Geometry: final body of the model. Coordinates: model frame, mm. A direction names the side the tool comes from. Round coordinates to 2 decimals unless told otherwise and drop trailing zeros. Write each loop counter-clockwise with the first axis right and the second up, starting at its lowest first coordinate (ties: lowest second). Pieces come first, ordered by that corner, then holes. Notation, with made-up numbers: (-24.5, 85) -> (-6.5, 85) arc R28 cw to (-6.5, 116) -> close; hole circle Ø6 at (31, 16). An arc over 180 degrees is marked (long way). One line per item, written item: value. Start each with the question number.
from build123d import *

# Parameters (mm, degrees)
F1_DEPTH = 50.8
F2_W     = 8.89
F2_H     = 8.255
F3_DEPTH = 38.1
F4_R     = 3.3655
F4_R_2   = 2.0955
F5_DEPTH = 2.54
F6_DEPTH = 53.34


with BuildPart() as f1:
    # F0 (on Top) → F1 (new body)
    with BuildSketch(Plane.XY):
        with BuildLine():
            Line((-27.305, 3.3655), (-27.305, 4.9141779831))
            ThreePointArc((-27.305, 4.9141779831), (-29.1268062902, -3.7268062902), (-20.4858220169, -1.905))
            Line((-20.4858220169, -1.905), (-22.0345, -1.905))
            Line((-22.0345, -1.905), (-22.0345, 0))
            ThreePointArc((-22.0345, 0), (-27.7797678721, -2.3797678721), (-25.4, 3.3655))
            Line((-25.4, 3.3655), (-27.305, 3.3655))
        make_face()
        with BuildLine():
            ThreePointArc((-23.495, 35.7206557626), (-25.4, 35.052), (-27.305, 35.7206557626))
            Line((-27.305, 35.7206557626), (-27.305, 4.9141779831))
            ThreePointArc((-27.305, 4.9141779831), (-25.4, 5.2705), (-23.495, 4.9141779831))
            Line((-23.495, 4.9141779831), (-23.495, 35.7206557626))
        make_face()
        with BuildLine():
            ThreePointArc((-23.495, 4.9141779831), (-25.4, 5.2705), (-27.305, 4.9141779831))
            Line((-27.305, 4.9141779831), (-27.305, 3.3655))
            Line((-27.305, 3.3655), (-25.4, 3.3655))
            Line((-25.4, 3.3655), (-23.495, 3.3655))
            Line((-23.495, 3.3655), (-23.495, 4.9141779831))
        make_face()
        with BuildLine():
            Line((-22.0345, -1.905), (-20.4858220169, -1.905))
            ThreePointArc((-20.4858220169, -1.905), (-20.2193463101, -0.9690188826), (-20.1295, 0))
            ThreePointArc((-20.1295, 0), (-20.2193463101, 0.9690188826), (-20.4858220169, 1.905))
            Line((-20.4858220169, 1.905), (-22.0345, 1.905))
            Line((-22.0345, 1.905), (-22.0345, 0))
            Line((-22.0345, 0), (-22.0345, -1.905))
        make_face()
        with BuildLine():
            ThreePointArc((-20.4858220169, 1.905), (-21.6731937098, 3.7268062902), (-23.495, 4.9141779831))
            Line((-23.495, 4.9141779831), (-23.495, 3.3655))
            Line((-23.495, 3.3655), (-25.4, 3.3655))
            ThreePointArc((-25.4, 3.3655), (-23.0202321279, 2.3797678721), (-22.0345, 0))
            Line((-22.0345, 0), (-22.0345, 1.905))
            Line((-22.0345, 1.905), (-20.4858220169, 1.905))
        make_face()
        with BuildLine():
            ThreePointArc((-20.1295, 0), (-20.2193463101, -0.9690188826), (-20.4858220169, -1.905))
            Line((-20.4858220169, -1.905), (0, -1.905))
            Line((0, -1.905), (0, 0))
            Line((0, 0), (0, 1.905))
            Line((0, 1.905), (-20.4858220169, 1.905))
            ThreePointArc((-20.4858220169, 1.905), (-20.2193463101, 0.9690188826), (-20.1295, 0))
        make_face()
        with BuildLine():
            Line((20.4858220169, 1.905), (0, 1.905))
            Line((0, 1.905), (0, 0))
            Line((0, 0), (20.1295, 0))
            ThreePointArc((20.1295, 0), (20.2193463101, 0.9690188826), (20.4858220169, 1.905))
        make_face()
        with BuildLine():
            Line((22.0345, 1.905), (20.4858220169, 1.905))
            ThreePointArc((20.4858220169, 1.905), (20.2193463101, 0.9690188826), (20.1295, 0))
            Line((20.1295, 0), (22.0345, 0))
            Line((22.0345, 0), (22.0345, 1.905))
        make_face()
        with BuildLine():
            Line((22.0345, -1.905), (20.4858220169, -1.905))
            ThreePointArc((20.4858220169, -1.905), (26.3690188826, -5.1806536899), (30.6705, 0))
            ThreePointArc((30.6705, 0), (29.7484751782, 2.9780755321), (27.305, 4.9141779831))
            Line((27.305, 4.9141779831), (27.305, 3.3655))
            Line((27.305, 3.3655), (25.4, 3.3655))
            ThreePointArc((25.4, 3.3655), (27.7797678721, 2.3797678721), (28.7655, 0))
            ThreePointArc((28.7655, 0), (25.4, -3.3655), (22.0345, 0))
            Line((22.0345, 0), (22.0345, -1.905))
        make_face()
        with BuildLine():
            ThreePointArc((20.1295, 0), (20.2193463101, -0.9690188826), (20.4858220169, -1.905))
            Line((20.4858220169, -1.905), (22.0345, -1.905))
            Line((22.0345, -1.905), (22.0345, 0))
            Line((22.0345, 0), (20.1295, 0))
        make_face()
        with BuildLine():
            Line((0, 0), (0, -1.905))
            Line((0, -1.905), (20.4858220169, -1.905))
            ThreePointArc((20.4858220169, -1.905), (20.2193463101, -0.9690188826), (20.1295, 0))
            Line((20.1295, 0), (0, 0))
        make_face()
        with BuildLine():
            Line((27.305, 3.3655), (27.305, 4.9141779831))
            ThreePointArc((27.305, 4.9141779831), (26.3690188826, 5.1806536899), (25.4, 5.2705))
            Line((25.4, 5.2705), (25.4, 3.3655))
            Line((25.4, 3.3655), (27.305, 3.3655))
        make_face()
        with BuildLine():
            ThreePointArc((25.4, 5.2705), (26.3690188826, 5.1806536899), (27.305, 4.9141779831))
            Line((27.305, 4.9141779831), (27.305, 35.7206557626))
            ThreePointArc((27.305, 35.7206557626), (26.4094708427, 35.2240179733), (25.4, 35.052))
            Line((25.4, 35.052), (25.4, 5.2705))
        make_face()
        with BuildLine():
            Line((23.495, 35.7206557626), (23.495, 4.9141779831))
            ThreePointArc((23.495, 4.9141779831), (24.4309811174, 5.1806536899), (25.4, 5.2705))
            Line((25.4, 5.2705), (25.4, 35.052))
            ThreePointArc((25.4, 35.052), (24.3905291573, 35.2240179733), (23.495, 35.7206557626))
        make_face()
        with BuildLine():
            ThreePointArc((25.4, 5.2705), (24.4309811174, 5.1806536899), (23.495, 4.9141779831))
            Line((23.495, 4.9141779831), (23.495, 3.3655))
            Line((23.495, 3.3655), (25.4, 3.3655))
            Line((25.4, 3.3655), (25.4, 5.2705))
        make_face()
        with BuildLine():
            ThreePointArc((23.495, 4.9141779831), (21.6731937098, 3.7268062902), (20.4858220169, 1.905))
            Line((20.4858220169, 1.905), (22.0345, 1.905))
            Line((22.0345, 1.905), (22.0345, 0))
            ThreePointArc((22.0345, 0), (23.0202321279, 2.3797678721), (25.4, 3.3655))
            Line((25.4, 3.3655), (23.495, 3.3655))
            Line((23.495, 3.3655), (23.495, 4.9141779831))
        make_face()
    extrude(amount=F1_DEPTH)

    # F2 (on Right) → F3 (cut, symmetric)
    with BuildSketch(Plane.YZ):
        with Locations((31.2756557626, 4.1275)):
            Rectangle(F2_W, F2_H)
        with BuildLine():
            Line((4.9141779831, 50.8), (4.9141779831, 30.582289685))
            add(Edge.make_bspline(
                [(4.9141779831, 30.582289685), (16.0486069147, 30.9902963569), (19.3334478065, 33.025734419), (35.7206557626, 43.18)],
                knots=[8.6020682106, 8.6020682106, 8.6020682106, 8.6020682106, 42.9134576882, 42.9134576882, 42.9134576882, 42.9134576882], degree=3))
            Line((35.7206557626, 43.18), (35.7206557626, 50.8))
            Line((35.7206557626, 50.8), (4.9141779831, 50.8))
        make_face()
        with BuildLine():
            add(Edge.make_bspline(
                [(-5.2705, 30.48), (-1.1621300748, 30.48), (2.1227108169, 30.48), (4.9141779831, 30.582289685)],
                knots=[0, 0, 0, 0, 8.6020682106, 8.6020682106, 8.6020682106, 8.6020682106], degree=3))
            Line((4.9141779831, 30.582289685), (4.9141779831, 50.8))
            Line((4.9141779831, 50.8), (-5.2705, 50.8))
            Line((-5.2705, 50.8), (-5.2705, 30.48))
        make_face()
    extrude(amount=F3_DEPTH, both=True, mode=Mode.SUBTRACT)

    # F4 (on face) → F5 (join)
    with BuildSketch(Plane(origin=(0, 0, 0), x_dir=(1, 0, 0), z_dir=(0, 0, -1))):
        with Locations((-25.4, 0)):
            Circle(F4_R)
        with Locations((-25.4, 0)):
            Circle(F4_R_2, mode=Mode.SUBTRACT)
        with BuildLine():
            ThreePointArc((30.6705, 0), (26.3690188826, 5.1806536899), (20.4858220169, 1.905))
            ThreePointArc((20.4858220169, 1.905), (20.1295, 0), (20.4858220169, -1.905))
            ThreePointArc((20.4858220169, -1.905), (21.6731937098, -3.7268062902), (23.495, -4.9141779831))
            ThreePointArc((23.495, -4.9141779831), (25.4, -5.2705), (27.305, -4.9141779831))
            ThreePointArc((27.305, -4.9141779831), (29.7484751782, -2.9780755321), (30.6705, 0))
        make_face()
        with Locations((25.4, 0)):
            Circle(F4_R, mode=Mode.SUBTRACT)
        with Locations((25.4, 0)):
            Circle(F4_R)
        with Locations((25.4, 0)):
            Circle(F4_R_2, mode=Mode.SUBTRACT)
    extrude(amount=-F5_DEPTH)

    # F0 (on Top) → F6 (join)
    with BuildSketch(Plane.XY):
        with BuildLine():
            Line((-27.305, 38.1), (-27.305, 35.7206557626))
            ThreePointArc((-27.305, 35.7206557626), (-25.4, 35.052), (-23.495, 35.7206557626))
            Line((-23.495, 35.7206557626), (-23.495, 38.1))
            Line((-23.495, 38.1), (-27.305, 38.1))
        make_face()
        with BuildLine():
            ThreePointArc((-23.495, 35.7206557626), (-22.6525699281, 36.7801772846), (-22.352, 38.1))
            ThreePointArc((-22.352, 38.1), (-26.7198227154, 40.8474300719), (-27.305, 35.7206557626))
            Line((-27.305, 35.7206557626), (-27.305, 38.1))
            Line((-27.305, 38.1), (-23.495, 38.1))
            Line((-23.495, 38.1), (-23.495, 35.7206557626))
        make_face()
        with BuildLine():
            ThreePointArc((28.448, 38.1), (24.0801772846, 40.8474300719), (23.495, 35.7206557626))
            Line((23.495, 35.7206557626), (23.495, 38.1))
            Line((23.495, 38.1), (25.4, 38.1))
            Line((25.4, 38.1), (27.305, 38.1))
            Line((27.305, 38.1), (27.305, 35.7206557626))
            ThreePointArc((27.305, 35.7206557626), (28.1474300719, 36.7801772846), (28.448, 38.1))
        make_face()
        with BuildLine():
            ThreePointArc((25.4, 35.052), (26.4094708427, 35.2240179733), (27.305, 35.7206557626))
            Line((27.305, 35.7206557626), (27.305, 38.1))
            Line((27.305, 38.1), (25.4, 38.1))
            Line((25.4, 38.1), (25.4, 35.052))
        make_face()
        with BuildLine():
            Line((23.495, 38.1), (23.495, 35.7206557626))
            ThreePointArc((23.495, 35.7206557626), (24.3905291573, 35.2240179733), (25.4, 35.052))
            Line((25.4, 35.052), (25.4, 38.1))
            Line((25.4, 38.1), (23.495, 38.1))
        make_face()
    extrude(amount=F6_DEPTH)


solid = f1.part
(1) Section query A-A (z = 11). Output: boundary loops of the cut face in (x, y) (1 decimal), and give its area (3 significant figures).
(2) Pull-direction query (Y, two-part tool) for faces 1 (the face through (4, 1, 0)), 2 (the face through (-25, 31, 8.255)), 3 (the face through (23.495, 21, 21)), 4 (the face through (0, -1.905, 15)); classes: pulls with the +Y half, pulls with the -Y half, needs draft (parallel to the pull), parting line crosses it, or undercut.
(3) Line query: probe 1 along X at (y, z) = (0, 0.9); probe 2 along Y at (x, z) = (-25.4, 1.7); probe 3 along X at (y, z) = (0, 14). Output: solid intervals per line, ascending.
(4) Set-up query: faces 5 (the face through (27, -2, 2.54)), 6 (the face through (27.305, 20, 21)), 7 (the face through (25, 26.831, 4)). Return all of +Z, -Z, +X, -X, +Y, -Y with unobstructed straight access to the full face (end or side cutting, diameter ignored); none if empty.
(5) Section query B-B (y = 36.5). Output: boundary loops of the cut face in (x, z), and give its area (3 significant figures).
(6) Pin query (flat end, axial travel): pin 1 (1.5 mm diameter, centred on x = 22.5, z = 36, fed in from +Y); pin 2 (8 mm diameter, centred on x = 13.5, z = 29, fed in from -Y) (3 decimals); pin 3 (4 mm diameter, centred on y = 12, z = 11.5, fed in from +X) (3 decimals); pin 4 (4 mm diameter, centred on x = -25, z = 5, fed in from +Y). Return the tip coordinate at first contact, or that it passes through.
Results list:
1. outline: (-27.3, 4.9) arc R5.3 ccw (long way) to (-20.5, -1.9) -> (20.5, -1.9) arc R5.3 ccw (long way) to (27.3, 4.9) -> (27.3, 35.7) arc R3 ccw (long way) to (23.5, 35.7) -> (23.5, 4.9) arc R5.3 ccw to (20.5, 1.9) -> (-20.5, 1.9) arc R5.3 ccw to (-23.5, 4.9) -> (-23.5, 35.7) arc R3 ccw (long way) to (-27.3, 35.7) -> close; hole circle Ø6.7 at (-25.4, 0); hole circle Ø6.7 at (25.4, 0)
1. area: 545 mm^2
2. face 1: needs draft
2. face 2: undercut
2. face 3: undercut
2. face 4: pulls with the -Y half
3. probe 1: x = -30.67 to -27.5, -23.3 to 23.3, 27.5 to 30.67
3. probe 2: y = -5.27 to -2.1, 2.1 to 26.83, 35.05 to 41.15
3. probe 3: x = -30.67 to -28.77, -22.03 to 22.03, 28.77 to 30.67
4. face 5: +Z
4. face 6: +Z, -Z, +X
4. face 7: -Z, +X, -X
5. outline: (-27.99, 0) -> (-22.81, 0) -> (-22.81, 53.34) -> (-27.99, 53.34) -> close; (22.81, 0) -> (27.99, 0) -> (27.99, 53.34) -> (22.81, 53.34) -> close
5. area: 554 mm^2
6. pin 1: stops at y = 40.26
6. pin 2: stops at y = -1.905
6. pin 3: stops at x = 27.305
6. pin 4: stops at y = 41.15
